```python
from build123d import *

# Parameters (mm, degrees)
SKETCH3_R           = 3.1
CUT_EXTRUDE1_DEPTH  = 222.614539842
BOSS_EXTRUDE1_START = 4
SKETCH4_R           = 49.000027987
SKETCH4_R_2         = 34.000027987
BOSS_EXTRUDE1_DEPTH = 4
CHAMFER1_SIZE       = 2
SKETCH5_R           = 1.5
BOSS_EXTRUDE2_DEPTH = 2


with BuildPart() as part:
    # Sketch2 → Revolve1 (revolve)
    with BuildSketch(Plane.XY, mode=Mode.PRIVATE) as revolve1_sk:
        with BuildLine():
            Line((340, 38.000027987), (300.010580524, 38.000027987))
            add(Edge.make_bspline(
                [(127, 23.368217816), (127.144658905, 23.387357923), (141.067067172, 25.227802685), (169.534203287, 28.668411554), (205.200950651, 32.237503735), (234.354838071, 34.660219308), (256.239727532, 36.200460456), (274.483617298, 37.216214614), (289.091810146, 37.788845449), (296.367863688, 37.980756791), (300.010580524, 38.000027987)],
                knots=[0.426924824, 0.426924824, 0.426924824, 0.426924824, 0.428368468, 0.565862687, 0.710575124, 0.782931343, 0.855287562, 0.927643781, 0.963821891, 1, 1, 1, 1], degree=3))
            Line((127, 23.368217816), (127, 0))
            Line((127, 0), (131, 0))
            Line((131, 0), (131, 20))
            ThreePointArc((131, 20), (215.320786735, 29.227370129), (300.010580524, 34.000027987))
            Line((300.010580524, 34.000027987), (340, 34.000027987))
            Line((340, 34.000027987), (340, 38.000027987))
        make_face()
    revolve(revolve1_sk.sketch.rotate(Axis((0, 0, 0), (1, 0, 0)), 90), axis=Axis((0, 0, 0), (1, 0, 0)))

    # Sketch3 → Cut-Extrude1 (cut, through all)
    with BuildSketch(Plane.ZY.offset(-125)):
        Circle(SKETCH3_R)
    extrude(amount=-CUT_EXTRUDE1_DEPTH, mode=Mode.SUBTRACT)

    # Sketch4 → Boss-Extrude1 (add)
    with BuildSketch(Plane(origin=(340, 0, 0), x_dir=(0, 0, -1), z_dir=(1, 0, 0)).offset(BOSS_EXTRUDE1_START)):
        Circle(SKETCH4_R)
        with Locations(Location((0, 0, 0), (0, 0, 180))):
            Circle(SKETCH4_R_2, mode=Mode.SUBTRACT)
    extrude(amount=-BOSS_EXTRUDE1_DEPTH)

    # Chamfer1
    chamfer1_edges = [part.edges().sort_by_distance(p)[0] for p in [
        (344, 0, -34.000027987),
    ]]
    chamfer(chamfer1_edges, length=CHAMFER1_SIZE)

    # Sketch5 → Boss-Extrude2 (add)
    with BuildSketch(Plane.ZY.offset(-127)):
        with Locations((0, 15)):
            Circle(SKETCH5_R)
        with Locations((15, 0)):
            Circle(SKETCH5_R)
        with Locations((-15, 0)):
            Circle(SKETCH5_R)
        with Locations((0, -15)):
            Circle(SKETCH5_R)
    extrude(amount=BOSS_EXTRUDE2_DEPTH)


solid = part.part
```
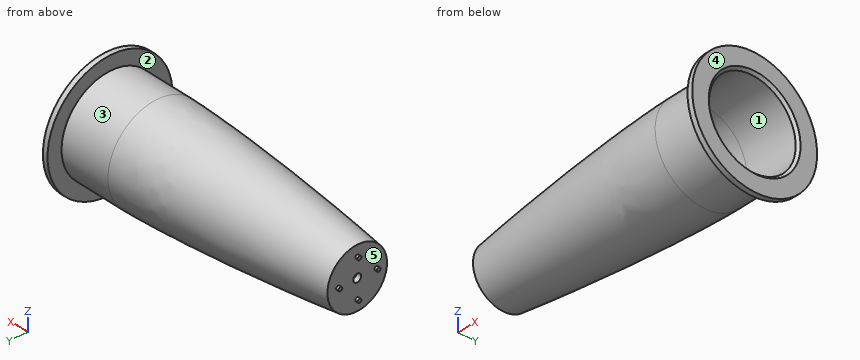
The listing builds one solid part. Answer for the finished solid, in the listing's coordinates (mm). Face numbers are marked on the shaded views. A direction names the side the tool comes from. Round coordinates to 2 decimals unless told otherwise and drop trailing zeros.
1) Given P1, Ø14, axis at y = 0, z = -4.5, coming from the -X side; P2, Ø4, axis at x = 307, y = -30, coming from the +Z side; P3, Ø4, axis at x = 189, z = 34, coming from the +Y side; P4, Ø5, axis at x = 310, y = 12, coming from the -Z side, each flat-ended and moving along its own axis, determine where each tip first touches the part or whether it passes through.
Outcome:
P1: stops at x = 127
P2: stops at z = 25.69
P3: passes through
P4: stops at z = -36.79
2) Consider line 1 (Y direction, x = 317, z = 0); line 2 (X direction, y = 16.5, z = -5); line 3 (X direction, y = -42.5, z = -0.5). Determine where each line is inside the solid, lowest interval first.
Outcome:
line 1: y = -38 to -34, 34 to 38
line 2: x = 127 to 131
line 3: x = 340 to 344
3) For the marked faces 4 and 5, determine the directions among +Z, -Z, +X, -X, +Y, -Y from which every point of the face is accessible in a straight line to the end or side of a thin tool.
Outcome:
face 4: +Z, -Z, +X, +Y, -Y
face 5: -X
4) For a pull along Y with two mould halves and no side action, classify the marked faces 1, 2 and 3 as released by +Y, released by -Y, zero draft, split by the parting line, or undercut.
Outcome:
face 1: undercut
face 2: zero draft
face 3: split by the parting line
